```python
from build123d import *

# Parameters (mm, degrees)
SKETCH2_W               = 101.6
SKETCH2_H               = 101.6
BOSS_EXTRUDE1_DEPTH     = 203.2
SKETCH4_W               = 88.9
SKETCH4_H               = 88.9
CUT_EXTRUDE1_DEPTH      = 95.25
FILLET1_R               = 12.7
SKETCH5_R               = 12.7
CUT_EXTRUDE2_DEPTH      = 102.6
SKETCH6_R               = 12.7
CUT_EXTRUDE3_DEPTH      = 102.6
CUT_EXTRUDE4_DEPTH      = 7.35
SKETCH31_W              = 22.86
SKETCH31_H              = 8.89
BOSS_EXTRUDE2_DEPTH     = 25.4
FILLET5_R               = 12.7
FILLET6_R               = 6.35
SKETCH38_R              = 4.953
CUT_EXTRUDE7_DEPTH      = 50.022
CUT_EXTRUDE7_DEPTH_BACK = 53.578


with BuildPart() as part:
    # Sketch2 → Boss-Extrude1 (new body)
    with BuildSketch(Plane(origin=(0, 0, 0), x_dir=(1, 0, 0), z_dir=(0, 1, 0))):
        with Locations((9.448577681, 25.677899344)):
            Rectangle(SKETCH2_W, SKETCH2_H)
    extrude(amount=BOSS_EXTRUDE1_DEPTH)

    # Sketch4 → Cut-Extrude1 (cut, symmetric)
    with BuildSketch(Plane(origin=(0, 101.6, 0), x_dir=(1, 0, 0), z_dir=(0, 1, 0))):
        with Locations((3.098577681, 32.027899344)):
            Rectangle(SKETCH4_W, SKETCH4_H)
    extrude(amount=CUT_EXTRUDE1_DEPTH, both=True, mode=Mode.SUBTRACT)

    # Fillet1
    fillet1_edges = [part.edges().sort_by_distance(p)[0] for p in [
        (47.548577681, 101.6, 12.422100656),
        (60.248577681, 101.6, 25.122100656),
    ]]
    fillet(fillet1_edges, radius=FILLET1_R)

    # Sketch5 → Cut-Extrude2 (cut, through all)
    with BuildSketch(Plane.XY.offset(25.122100656)):
        with Locations((-3.251422319, 177.8)):
            Circle(SKETCH5_R)
        with Locations((-3.251422319, 139.7)):
            Circle(SKETCH5_R)
        with Locations((-3.251422319, 101.6)):
            Circle(SKETCH5_R)
        with Locations((-3.251422319, 63.5)):
            Circle(SKETCH5_R)
        with Locations((-3.251422319, 25.4)):
            Circle(SKETCH5_R)
    extrude(amount=-CUT_EXTRUDE2_DEPTH, mode=Mode.SUBTRACT)

    # Sketch6 → Cut-Extrude3 (cut, through all)
    with BuildSketch(Plane(origin=(60.248577681, 0, 0), x_dir=(0, 0, -1), z_dir=(1, 0, 0))):
        with Locations((38.377899344, 177.8)):
            Circle(SKETCH6_R)
        with Locations((38.377899344, 139.7)):
            Circle(SKETCH6_R)
        with Locations((38.377899344, 101.6)):
            Circle(SKETCH6_R)
        with Locations((38.377899344, 63.5)):
            Circle(SKETCH6_R)
        with Locations((38.377899344, 25.4)):
            Circle(SKETCH6_R)
    extrude(amount=-CUT_EXTRUDE3_DEPTH, mode=Mode.SUBTRACT)

    # Sketch7 → Cut-Extrude4 (cut, through all)
    with BuildSketch(Plane(origin=(0, 6.35, 0), x_dir=(1, 0, 0), z_dir=(0, 1, 0))):
        with BuildLine():
            Line((-41.351422319, 76.477899344), (47.548577681, 76.477899344))
            Line((47.548577681, 76.477899344), (47.548577681, 0.277899344))
            ThreePointArc((47.548577681, 0.277899344), (43.828833802, -8.702356778), (34.848577681, -12.422100656))
            Line((34.848577681, -12.422100656), (-41.351422319, -12.422100656))
            Line((-41.351422319, -12.422100656), (-41.351422319, 76.477899344))
        make_face()
    extrude(amount=-CUT_EXTRUDE4_DEPTH, mode=Mode.SUBTRACT)

    # Sketch31 → Boss-Extrude2 (add)
    with BuildSketch(Plane.XZ.offset(-196.85)):
        with Locations((-29.921422319, -2.182899344)):
            Rectangle(SKETCH31_W, SKETCH31_H)
        with Locations((-29.921422319, -23.010899344)):
            Rectangle(SKETCH31_W, SKETCH31_H)
    extrude(amount=BOSS_EXTRUDE2_DEPTH)

    # Fillet5
    fillet5_edges = [part.edges().sort_by_distance(p)[0] for p in [
        (-41.351422319, 171.45, -2.182899344),
        (-41.351422319, 171.45, -23.010899344),
    ]]
    fillet(fillet5_edges, radius=FILLET5_R)

    # Fillet6
    fillet6_edges = [part.edges().sort_by_distance(p)[0] for p in [
        (-18.491422319, 171.45, -2.182899344),
        (-18.491422319, 171.45, -23.010899344),
    ]]
    fillet(fillet6_edges, radius=FILLET6_R)

    # Sketch38 → Cut-Extrude7 (cut, two sides)
    with BuildSketch(Plane(origin=(0, 0, -27.455899344), x_dir=(-1, 0, 0), z_dir=(0, 0, -1))) as cut_extrude7_sk:
        with Locations((29.286422319, 184.023)):
            Circle(SKETCH38_R)
    extrude(amount=CUT_EXTRUDE7_DEPTH, mode=Mode.SUBTRACT)
    extrude(cut_extrude7_sk.sketch, amount=-CUT_EXTRUDE7_DEPTH_BACK, mode=Mode.SUBTRACT)


solid = part.part
```
Here's how the part is built. I have some questions about the finished solid (model axes, mm). A direction names the side the tool comes from. Give positions to 0.01 mm unless a question says otherwise; leave off trailing zeros. Write each loop counter-clockwise with the first axis right and the second up, starting at its lowest first coordinate (ties: lowest second). Pieces come first, ordered by that corner, then holes. Notation, with made-up numbers: M -21.5,-38 L 14.5,-38 A19 ccw 14.5,-12 Z; hole C -11.5,2.25 d2. An arc over 180 degrees is marked long. Put each result on its own line as item: value. Start each with the question number.
Item 1: Will these pins go through, and if not, where does the flat tip stop? pin 1 (5 mm diameter, centred on x = 15.5, z = -33, fed in from -Y); pin 2 (1.1 mm diameter, centred on x = -26.5, z = -21, fed in from -Y); pin 3 (4 mm diameter, centred on y = 134, z = -4.5, fed in from -X).
Item 2: I need wall thicknesses on L1, parallel to Y at x = -2.5, z = 13.5; L2, parallel to Y at x = -0.5, z = 16; L3, parallel to X at y = 77, z = -53.5. Which ranges of each line are inside material? Lowest first, please. Write a range as from..to.
Item 3: If we section it at C-C, the plane z = -32.5: Write out the boundary of the cut face in (x, y), then the cut area to 3 significant figures.
Item 4: If we section it at A-A, the plane y = 63.5: Write out the boundary of the cut face in (x, z), then the cut area to 3 significant figures.
Item 5: On a 3-axis mill with a long thin cutter (end or side, diameter ignored), from which of +Z, -Z, +X, -X, +Y, -Y can I reach the whole of each face in a straight line? I mean faces 4 (the cylindrical face through (-4.905, 152.292, 18.861)), 5 (the flat face through (9, 203.2, -26)), 6 (the cylindrical face through (-20.4, 173.26, -22.95)), 7 (the flat face through (-27, 171.45, -2)), 8 (the flat face through (-30, 190, 2.262)). Say none if no direction works.
Item 6: If we section it at B-B, the plane x = 3.5: Write out the boundary of the cut face in (y, z), then the cut area to 3 significant figures.
Item 7: Thinking about a two-plate mould opening in Y: for faces 1 (the flat face through (2, 196.85, -33)), 2 (the flat face through (-18.491, 187, -2)), 3 (the cylindrical face through (53.99, 114.19, -36.72)), which applies, +Y half, -Y half, draft (parallel to the pull), parting line (faces both ways), or undercut?
Item 8: If we section it at D-D, the plane y = 175.5: Write out the boundary of the cut face in (x, z).
Values:
1. pin 1: y = 196.85
1. pin 2: y = 171.45
1. pin 3: x = 47.55
2. L1: 0..12.72, 38.08..50.82, 76.18..88.92, 114.28..127.02, 152.38..165.12, 190.48..203.2
2. L2: 0..13, 37.8..51.1, 75.9..89.2, 114..127.3, 152.1..165.4, 190.2..203.2
2. L3: 47.55..60.25
3. outline: M -41.35,196.85 L 47.55,196.85 L 47.55,189.06 L 60.25,189.06 L 60.25,203.2 L -41.35,203.2 Z; M 47.55,0 L 60.25,0 L 60.25,14.14 L 47.55,14.14 Z; M 47.55,36.66 L 60.25,36.66 L 60.25,52.24 L 47.55,52.24 Z; M 47.55,74.76 L 60.25,74.76 L 60.25,90.34 L 47.55,90.34 Z; M 47.55,112.86 L 60.25,112.86 L 60.25,128.44 L 47.55,128.44 Z; M 47.55,150.96 L 60.25,150.96 L 60.25,166.54 L 47.55,166.54 Z
3. area: 1,720 mm²
4. outline: M -41.35,12.42 L -15.95,12.42 L -15.95,25.12 L -41.35,25.12 Z; M 9.45,12.42 L 34.85,12.42 A12.7 cw 47.55,-0.28 L 47.55,-25.68 L 60.25,-25.68 L 60.25,12.42 A12.7 ccw 47.55,25.12 L 9.45,25.12 Z; M 47.55,-76.48 L 60.25,-76.48 L 60.25,-51.08 L 47.55,-51.08 Z
4. area: 1,770 mm²
5. face 4: +Z, -Z
5. face 5: +Z, -Z, +X, -X, +Y
5. face 6: -Z, -Y
5. face 7: -Z, -X, -Y
5. face 8: -X, -Y
6. outline: M 0,12.42 L 14.64,12.42 L 14.64,25.12 L 0,25.12 Z; M 36.16,12.42 L 52.74,12.42 L 52.74,25.12 L 36.16,25.12 Z; M 74.26,12.42 L 90.84,12.42 L 90.84,25.12 L 74.26,25.12 Z; M 112.36,12.42 L 128.94,12.42 L 128.94,25.12 L 112.36,25.12 Z; M 150.46,12.42 L 167.04,12.42 L 167.04,25.12 L 150.46,25.12 Z; M 188.56,12.42 L 196.85,12.42 L 196.85,-76.48 L 203.2,-76.48 L 203.2,25.12 L 188.56,25.12 Z
6. area: 1,780 mm²
7. face 1: -Y half
7. face 2: draft
7. face 3: undercut
8. outline: M -41.35,12.42 L -15.74,12.42 L -15.74,25.12 L -41.35,25.12 Z; M -37.95,-27.46 L -18.92,-27.46 L -18.92,-18.57 L -37.95,-18.57 Z; M -37.95,-6.63 L -18.92,-6.63 L -18.92,2.26 L -37.95,2.26 Z; M 9.24,12.42 L 34.85,12.42 A12.7 cw 47.55,-0.28 L 47.55,-25.89 L 60.25,-25.89 L 60.25,12.42 A12.7 ccw 47.55,25.12 L 9.24,25.12 Z; M 47.55,-76.48 L 60.25,-76.48 L 60.25,-50.87 L 47.55,-50.87 Z
